Source: three-view drawing plus pictorial views. Frame: mm from the lowest corner of the part. Give positions to 0.01 mm unless a question says otherwise; leave off trailing zeros. Loops run counter-clockwise (first coordinate to the right, second up) from the corner with the lowest first, then second, coordinate; pieces in that order, holes last.
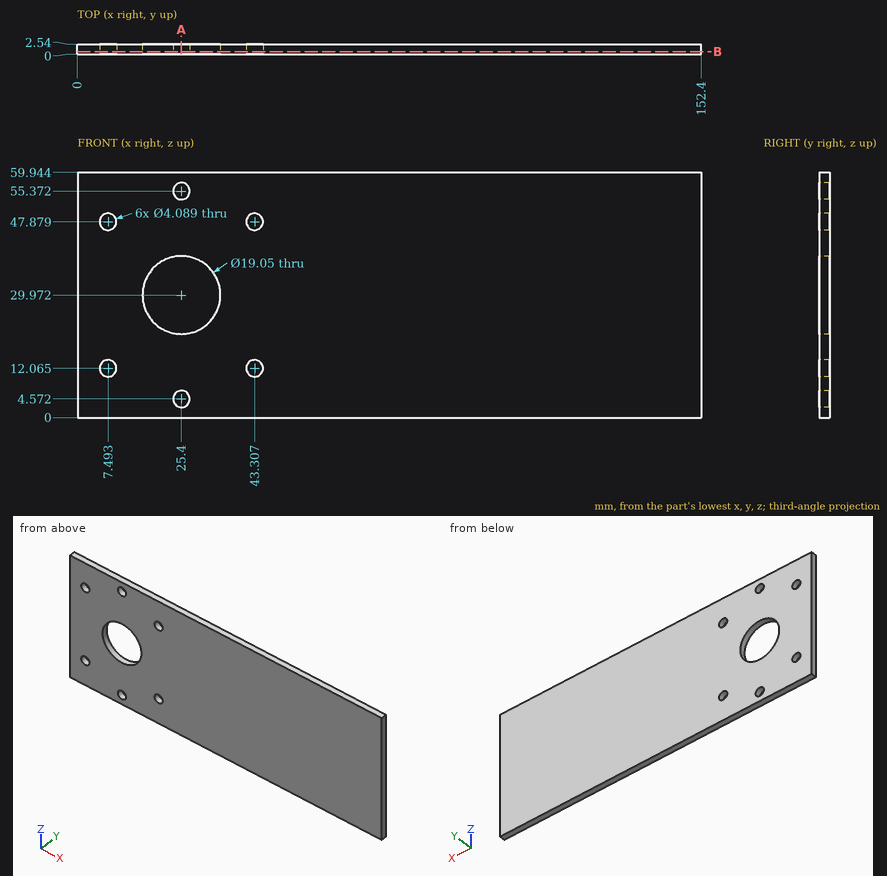
1) Ray query, probe 1 along X at (y, z) = (0.1, 4.5); probe 2 along X at (y, z) = (0.5, 46.5) (1 decimal); probe 3 along Z at (x, y) = (23, 2.1) (1 decimal). Return the intervals inside material, ascending.
Checks:
probe 1: x = 0 to 23.36, 27.44 to 152.4
probe 2: x = 0 to 6, 9 to 41.8, 44.8 to 152.4
probe 3: z = 0 to 20.8, 39.2 to 59.9
2) Cut plane B-B (y = 0.7). State how many separate pieces and enclosed holes the cut face has, and give its area (3 significant figures).
Checks:
separate pieces: 1
enclosed holes: 7
area: 8,770 mm2
3) Cut plane A-A (x = 25.4). Return loops of the section in (y, z).
Checks:
outline: (0, 0) - (2.54, 0) - (2.54, 2.53) - (0, 2.53) - close; (0, 6.62) - (2.54, 6.62) - (2.54, 20.45) - (0, 20.45) - close; (0, 39.5) - (2.54, 39.5) - (2.54, 53.33) - (0, 53.33) - close; (0, 57.42) - (2.54, 57.42) - (2.54, 59.94) - (0, 59.94) - close
4) Contact query for a flat-ended pin moving along its axis: P1, Ø6.5, axis at x = 25.4, z = 4.572, coming from the +Y side. Output: stop coordinate, or through.
Checks:
P1: stops at y = 2.54
